Study the drawing (mm; zero at the part's minimum x, y, z) and answer. Coordinates: 2 decimals unless noted, no trailing zeros. Order: outer loops, then holes, each group sorted by start corner. A loop starts at its lowest first (then second) coordinate and runs counter-clockwise, first axis right, second up.
1. The part is cut by section A-A, the plane z = 32.5. Give the vertices of the cut face in (x, y) (1 decimal), then the cut area to 3 significant figures.
2. Find the intervals of material crossed by probe 1 along X at (y, z) = (1.15, 63.5) (1 decimal); probe 2 along X at (y, z) = (1.25, 74); probe 3 along Z at (x, y) = (49.5, 0.3), in increasing order.
3. The part is cut by section C-C, the plane y = 2.7. Count the separate pieces of the cut face and the enclosed holes in it, then the cut area to 3 significant figures.
4. Flat-ended cylindrical pins translate along their axes: pin 1 Ø1.1 at (x, y) = (227, 2.5) entering from +Z; pin 2 Ø1.9 at (y, z) = (1.5, 84) entering from +X; pin 3 Ø1.9 at (y, z) = (2.5, 4) entering from -X. Find the tip coordinate at first contact, or state that the pin passes through.
5. The part is cut by section B-B, the plane x = 75. Give the vertices of the cut face in (y, z) (1 decimal).
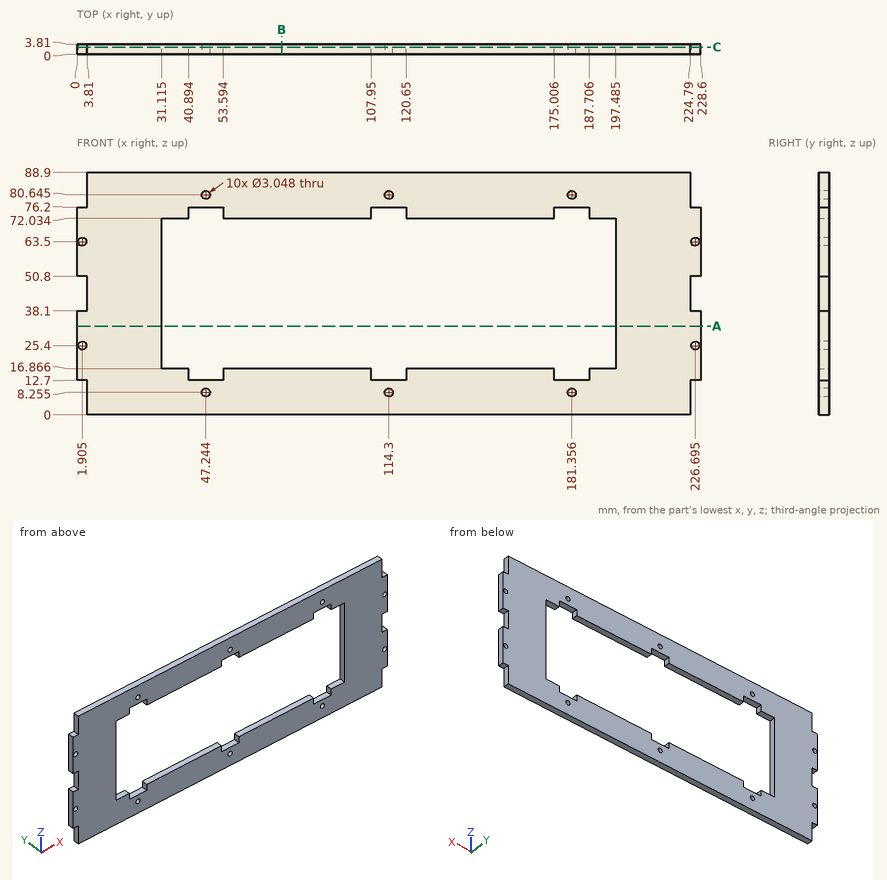
Geometry says:
1. outline: (0, 0) - (31.1, 0) - (31.1, 3.8) - (0, 3.8) - close; (197.5, 0) - (228.6, 0) - (228.6, 3.8) - (197.5, 3.8) - close
1. area: 237 mm2
2. probe 1: x = 0 to 0.4, 3.4 to 31.1, 197.5 to 225.2, 228.2 to 228.6
2. probe 2: x = 0 to 40.89, 53.59 to 107.95, 120.65 to 175.01, 187.71 to 228.6
2. probe 3: z = 0 to 12.7, 76.2 to 88.9
3. separate pieces: 1
3. enclosed holes: 11
3. area: 10,500 mm2
4. pin 1: stops at z = 76.2
4. pin 2: stops at x = 224.79
4. pin 3: stops at x = 3.81
5. outline: (0, 0) - (3.8, 0) - (3.8, 16.9) - (0, 16.9) - close; (0, 72) - (3.8, 72) - (3.8, 88.9) - (0, 88.9) - close
